Verification items for the finished model (mm, model axes). Face numbers are marked on the shaded views. A direction names the side the tool comes from. Round coordinates to 2 decimals unless told otherwise and drop trailing zeros. Loops run counter-clockwise (first coordinate to the right, second up) from the corner with the lowest first, then second, coordinate; pieces in that order, holes last. Notation, with made-up numbers: M 88.5,73.5 L 115.5,73.5 A11 ccw 115.5,81.5 Z; hole C -39,84.25 d9. An arc over 180 degrees is marked long. Answer as CSV lines item,"result".
```python
from build123d import *

# Parameters (mm, degrees)
CROQUIS1_R              = 5
CROQUIS1_R_2            = 1.95828143
SALIENTE_EXTRUIR1_DEPTH = 10
CROQUIS2_R              = 2.526447491
CROQUIS2_R_2            = 2.994638929
CORTAR_EXTRUIR1_DEPTH   = 45.283179651


with BuildPart() as part:
    # Croquis1 → Saliente-Extruir1 (new body)
    with BuildSketch(Plane(origin=(0, 0, 0), x_dir=(0, 0, -1), z_dir=(1, 0, 0))):
        Polygon((15, -31), (5, -31), (5, -16), (-5, -16), (-5, -31), (-15, -31), (-15, 31), (-5.542055275, 31), (-5.542055275, 16), (6.50834207, 16), (6.50834207, 31), (15, 31), align=None)
        Circle(CROQUIS1_R, mode=Mode.SUBTRACT)
        with Locations((-8, 0)):
            Circle(CROQUIS1_R_2, mode=Mode.SUBTRACT)
        with Locations((0, 8)):
            Circle(CROQUIS1_R_2, mode=Mode.SUBTRACT)
        with Locations((8, 0)):
            Circle(CROQUIS1_R_2, mode=Mode.SUBTRACT)
        with Locations((0, -8)):
            Circle(CROQUIS1_R_2, mode=Mode.SUBTRACT)
    extrude(amount=SALIENTE_EXTRUIR1_DEPTH)

    # Croquis2 → Cortar-Extruir1 (cut, through all)
    with BuildSketch(Plane.XY.offset(15)):
        with Locations((5, 25)):
            Circle(CROQUIS2_R)
        with Locations((5, -25)):
            Circle(CROQUIS2_R_2)
    extrude(amount=-CORTAR_EXTRUIR1_DEPTH, mode=Mode.SUBTRACT)


solid = part.part
```
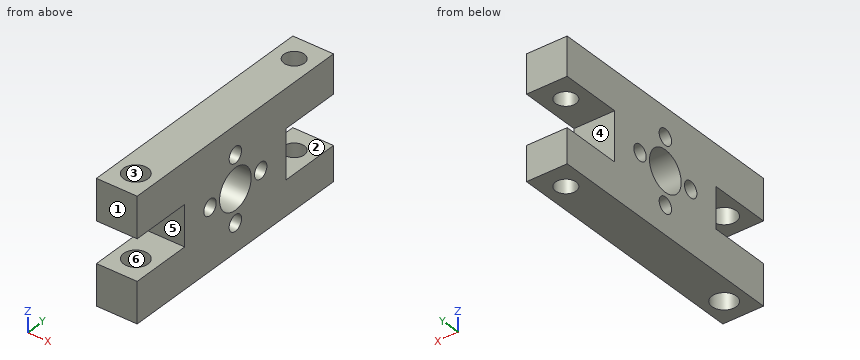
1) Section check C-C (y = -25). Record the cut outline in (x, z).
Here are the results:
outline,"M 0,-15 L 2.01,-15 L 2.01,-5 L 0,-5 Z; M 0,5 L 2.01,5 L 2.01,15 L 0,15 Z; M 7.99,-15 L 10,-15 L 10,-5 L 7.99,-5 Z; M 7.99,5 L 10,5 L 10,15 L 7.99,15 Z"
2) Section check A-A (z = 0). Record the cut outline in (x, y).
Here are the results:
outline,"M 0,-16 L 10,-16 L 10,-9.96 L 0,-9.96 Z; M 0,-6.04 L 10,-6.04 L 10,-5 L 0,-5 Z; M 0,5 L 10,5 L 10,6.04 L 0,6.04 Z; M 0,9.96 L 10,9.96 L 10,16 L 0,16 Z"
3) Set-up check for the marked faces 4, 5 and 6: record each of +Z, -Z, +X, -X, +Y, -Y from which the full face is reachable in a straight line by a thin tool's end or side.
Here are the results:
face 4,"+X, -X, +Y"
face 5,"+X, -X, -Y"
face 6,"+Z, -Z"
4) Material ranges on probe 1 along Y at (x, z) = (6.5, 0); probe 2 along Z at (x, y) = (1.25, 27.5); probe 3 along Z at (x, y) = (2, -21), recorded low to high.
Here are the results:
probe 1,"y = -16 to -9.96, -6.04 to -5, 5 to 6.04, 9.96 to 16"
probe 2,"z = -15 to -6.51, 5.54 to 15"
probe 3,"z = -15 to -5, 5 to 15"
5) Section check D-D (x = 9). Record the cut outline in (y, z), plus the area to 3 significant figures.
Here are the results:
outline,"M -31,-15 L 31,-15 L 31,-6.51 L 16,-6.51 L 16,5.54 L 31,5.54 L 31,15 L -31,15 L -31,5 L -16,5 L -16,-5 L -31,-5 Z; hole C -8,0 d3.92; hole C 0,0 d10; hole C 0,-8 d3.92; hole C 0,8 d3.92; hole C 8,0 d3.92"
area,"1,400 mm^2"
6) Draft check along Y on the marked faces 1, 2 and 3. Enter one of: +Y half, -Y half, draft (parallel to the pull), parting line (faces both ways), or undercut.
Here are the results:
face 1,"-Y half"
face 2,"draft"
face 3,"undercut"
7) Section check B-B (x = 5). State how many separate pieces and enclosed holes the cut face has, plus the area to 3 significant figures.
Here are the results:
separate pieces,"5"
enclosed holes,"5"
area,"1,190 mm^2"
8) Go/stop test with flat-tipped pins: pin 1 (3 mm diameter, centred on x = 7, z = -1, fed in from +Y); pin 2 (3 mm diameter, centred on x = 2.5, z = -1.5, fed in from -Y). Record where each tip stops, or that it passes through.
Here are the results:
pin 1,"stops at y = 16"
pin 2,"stops at y = -16"
